from build123d import *

# Parameters (mm, degrees)
SKETCH1_R             = 1.2192
BOSS_EXTRUDE1_DEPTH   = 3.1242
BOSS_EXTRUDE1_2_DEPTH = 3.1242
BOSS_EXTRUDE1_3_DEPTH = 3.1242
BOSS_EXTRUDE1_4_DEPTH = 3.1242
BOSS_EXTRUDE2_START   = -1.27
SKETCH2_R             = 1.2192
BOSS_EXTRUDE2_DEPTH   = 1.27
SKETCH4_W             = 5.9436
SKETCH4_H             = 1.27
CUT_EXTRUDE1_DEPTH    = 1.27
FILLET1_DEPTH         = 3.1242
FILLET1_START         = 1.8542
FILLET1_2_DEPTH       = 1.27
BOSS_EXTRUDE3_DEPTH   = 1.27
FILLET2_R             = 0.889
FILLET3_R             = 0.889
FILLET5_R             = 1.27


with BuildPart() as part:
    # Sketch1 → Boss-Extrude1 (new body)
    with BuildSketch(Plane(origin=(0, 0, 0), x_dir=(1, 0, 0), z_dir=(0, 1, 0))):
        with BuildLine():
            Line((26.2382, 18.587486955), (26.2382, 12.248113045))
            ThreePointArc((26.2382, 12.248113045), (30.9753, 15.4178), (26.2382, 18.587486955))
        make_face()
        with Locations(Location((28.67025, 15.4178, 0), (0, 0, 270))):
            Circle(SKETCH1_R, mode=Mode.SUBTRACT)
    extrude(amount=BOSS_EXTRUDE1_DEPTH)



with BuildPart() as body_2:
    # Sketch1 → Boss-Extrude1 2 (new body)
    with BuildSketch(Plane(origin=(0, 0, 0), x_dir=(1, 0, 0), z_dir=(0, 1, 0))):
        with BuildLine():
            Line((-26.2382, 18.587486955), (-26.2382, 12.248113045))
            ThreePointArc((-26.2382, 12.248113045), (-30.9753, 15.4178), (-26.2382, 18.587486955))
        make_face()
        with Locations(Location((-28.67025, 15.4178, 0), (0, 0, 270))):
            Circle(SKETCH1_R, mode=Mode.SUBTRACT)
    extrude(amount=BOSS_EXTRUDE1_2_DEPTH)


with BuildPart() as body_3:
    # Sketch1 → Boss-Extrude1 3 (new body)
    with BuildSketch(Plane(origin=(0, 0, 0), x_dir=(1, 0, 0), z_dir=(0, 1, 0))):
        with BuildLine():
            Line((26.2382, -12.248113045), (26.2382, -18.587486955))
            ThreePointArc((26.2382, -18.587486955), (30.9753, -15.4178), (26.2382, -12.248113045))
        make_face()
        with Locations(Location((28.67025, -15.4178, 0), (0, 0, 270))):
            Circle(SKETCH1_R, mode=Mode.SUBTRACT)
    extrude(amount=BOSS_EXTRUDE1_3_DEPTH)


with BuildPart() as body_4:
    # Sketch1 → Boss-Extrude1 4 (new body)
    with BuildSketch(Plane(origin=(0, 0, 0), x_dir=(1, 0, 0), z_dir=(0, 1, 0))):
        with BuildLine():
            Line((-26.2382, -12.248113045), (-26.2382, -18.587486955))
            ThreePointArc((-26.2382, -18.587486955), (-30.9753, -15.4178), (-26.2382, -12.248113045))
        make_face()
        with Locations(Location((-28.67025, -15.4178, 0), (0, 0, 270))):
            Circle(SKETCH1_R, mode=Mode.SUBTRACT)
    extrude(amount=BOSS_EXTRUDE1_4_DEPTH)


with BuildPart() as part_1:
    add(part.part)

    add(body_2.part)  # Boss-Extrude2 merges body 2

    add(body_3.part)  # Boss-Extrude2 merges body 3

    add(body_4.part)  # Boss-Extrude2 merges body 4
    # Sketch2 → Boss-Extrude2 (add)
    with BuildSketch(Plane(origin=(0, 3.1242, 0), x_dir=(1, 0, 0), z_dir=(0, 1, 0)).offset(BOSS_EXTRUDE2_START)):
        with BuildLine():
            Line((-24.695157071, 17.3228), (24.695157071, 17.3228))
            ThreePointArc((24.695157071, 17.3228), (30.864949116, 16.280707319), (25.9842, 12.365278978))
            Line((25.9842, 12.365278978), (25.9842, -12.365278978))
            ThreePointArc((25.9842, -12.365278978), (30.879851828, -14.614386528), (27.5463, -18.8468))
            Line((27.5463, -18.8468), (-27.5463, -18.8468))
            ThreePointArc((-27.5463, -18.8468), (-30.879851828, -14.614386528), (-25.9842, -12.365278978))
            Line((-25.9842, -12.365278978), (-25.9842, 12.365278978))
            ThreePointArc((-25.9842, 12.365278978), (-30.864949116, 16.280707319), (-24.695157071, 17.3228))
        make_face()
        with Locations(Location((28.67025, -15.4178, 0), (0, 0, 270))):
            Circle(SKETCH2_R, mode=Mode.SUBTRACT)
        with Locations(Location((28.67025, 15.4178, 0), (0, 0, 270))):
            Circle(SKETCH2_R, mode=Mode.SUBTRACT)
        with Locations(Location((-28.67025, 15.4178, 0), (0, 0, 270))):
            Circle(SKETCH2_R, mode=Mode.SUBTRACT)
        with Locations(Location((-28.67025, -15.4178, 0), (0, 0, 270))):
            Circle(SKETCH2_R, mode=Mode.SUBTRACT)
    extrude(amount=BOSS_EXTRUDE2_DEPTH)

    # Sketch4 → Cut-Extrude1 (cut)
    with BuildSketch(Plane(origin=(0, 3.1242, 0), x_dir=(1, 0, 0), z_dir=(0, 1, 0))):
        with Locations((-10.8458, -18.2118)):
            Rectangle(SKETCH4_W, SKETCH4_H)
    extrude(amount=-CUT_EXTRUDE1_DEPTH, mode=Mode.SUBTRACT)

    # Fillet1: read off the stored shape, not the designer's step
    # Fillet1 outline → Fillet1 (add)
    with BuildSketch(Plane(origin=(0, 0, 0), x_dir=(1, 0, 0), z_dir=(0, 1, 0))):
        with BuildLine():
            Line((26.2382, 12.248113045), (26.2382, 9.318072184))
            ThreePointArc((26.2382, 9.318072184), (27.272818982, 11.08465566), (28.933486364, 12.281918148))
            ThreePointArc((28.933486364, 12.281918148), (27.58930418, 11.989069675), (26.2382, 12.248113045))
        make_face()
        with BuildLine():
            ThreePointArc((28.933486364, -12.281918148), (27.272818982, -11.08465566), (26.2382, -9.318072184))
            Line((26.2382, -9.318072184), (26.2382, -12.248113045))
            ThreePointArc((26.2382, -12.248113045), (27.58930418, -11.989069675), (28.933486364, -12.281918148))
        make_face()
        with BuildLine():
            Line((-26.2382, 9.318072184), (-26.2382, 12.248113045))
            ThreePointArc((-26.2382, 12.248113045), (-27.58930418, 11.989069675), (-28.933486364, 12.281918148))
            ThreePointArc((-28.933486364, 12.281918148), (-27.272818982, 11.08465566), (-26.2382, 9.318072184))
        make_face()
        with BuildLine():
            Line((-26.2382, -12.248113045), (-26.2382, -9.318072184))
            ThreePointArc((-26.2382, -9.318072184), (-27.272818982, -11.08465566), (-28.933486364, -12.281918148))
            ThreePointArc((-28.933486364, -12.281918148), (-27.58930418, -11.989069675), (-26.2382, -12.248113045))
        make_face()
    extrude(amount=FILLET1_DEPTH)

    # Fillet1 2 outline → Fillet1 2 (add)
    with BuildSketch(Plane(origin=(0, 0, 0), x_dir=(1, 0, 0), z_dir=(0, 1, 0)).offset(FILLET1_START)):
        with BuildLine():
            ThreePointArc((25.9842, 7.752311027), (26.048112355, 8.545425773), (26.2382, 9.318072184))
            Line((26.2382, 9.318072184), (26.2382, 12.248113045))
            ThreePointArc((26.2382, 12.248113045), (26.110004775, 12.304104924), (25.9842, 12.365278978))
            Line((25.9842, 12.365278978), (25.9842, 7.752311027))
        make_face()
        with BuildLine():
            ThreePointArc((26.2382, -9.318072184), (26.048112355, -8.545425773), (25.9842, -7.752311027))
            Line((25.9842, -7.752311027), (25.9842, -12.365278978))
            ThreePointArc((25.9842, -12.365278978), (26.110004775, -12.304104924), (26.2382, -12.248113045))
            Line((26.2382, -12.248113045), (26.2382, -9.318072184))
        make_face()
        with BuildLine():
            Line((-25.9842, -12.365278978), (-25.9842, -7.752311027))
            ThreePointArc((-25.9842, -7.752311027), (-26.048112355, -8.545425773), (-26.2382, -9.318072184))
            Line((-26.2382, -9.318072184), (-26.2382, -12.248113045))
            ThreePointArc((-26.2382, -12.248113045), (-26.110004775, -12.304104924), (-25.9842, -12.365278978))
        make_face()
        with BuildLine():
            Line((-24.695157071, 17.3228), (-22.726988846, 17.3228))
            ThreePointArc((-22.726988846, 17.3228), (-24.220374536, 17.553299795), (-25.574763619, 18.223345455))
            ThreePointArc((-25.574763619, 18.223345455), (-25.093280542, 17.813783418), (-24.695157071, 17.3228))
        make_face()
        with BuildLine():
            ThreePointArc((24.695157071, 17.3228), (25.093280542, 17.813783418), (25.574763619, 18.223345455))
            ThreePointArc((25.574763619, 18.223345455), (24.220374536, 17.553299795), (22.726988846, 17.3228))
            Line((22.726988846, 17.3228), (24.695157071, 17.3228))
        make_face()
        with BuildLine():
            ThreePointArc((-25.9842, 12.365278978), (-26.110004775, 12.304104924), (-26.2382, 12.248113045))
            Line((-26.2382, 12.248113045), (-26.2382, 9.318072184))
            ThreePointArc((-26.2382, 9.318072184), (-26.048112355, 8.545425773), (-25.9842, 7.752311027))
            Line((-25.9842, 7.752311027), (-25.9842, 12.365278978))
        make_face()
    extrude(amount=FILLET1_2_DEPTH)

    # Sketch7 → Boss-Extrude3 (add)
    with BuildSketch(Plane(origin=(0, 3.1242, 0), x_dir=(1, 0, 0), z_dir=(0, 1, 0))):
        Polygon((-7.874, -25.0444), (-7.874, -35.3314), (23.9649, -35.3314), (23.9649, -25.0444), (23.9649, -18.8468), (-7.874, -18.8468), align=None)
    extrude(amount=-BOSS_EXTRUDE3_DEPTH)

    # Fillet2
    fillet2_edges = [part_1.edges().sort_by_distance(p)[0] for p in [
        (-13.8176, 2.4892, 17.5768),
        (-7.874, 2.4892, 17.5768),
        (23.9649, 2.4892, 18.8468),
    ]]
    fillet(fillet2_edges, radius=FILLET2_R)

    # Fillet3
    fillet3_edges = [part_1.edges().sort_by_distance(p)[0] for p in [
        (-13.8176, 2.4892, 18.8468),
        (23.9649, 2.4892, 35.3314),
        (-7.874, 2.4892, 35.3314),
    ]]
    fillet(fillet3_edges, radius=FILLET3_R)

    # Fillet5
    # the kernel refuses this fillet: 1.27 mm, written as the material it takes off along each edge
    with BuildSketch(Plane(origin=(26.2382, -9.068202779, -9.318072184), x_dir=(0, 0, -1), z_dir=(0, 1, 0)), Plane(origin=(-26.2382, -9.068202779, 9.318072184), x_dir=(0, 0, 1), z_dir=(0, 1, 0))) as fillet5_piece_1:
        with BuildLine():
            CenterArc((3.627281111, -1.27), FILLET5_R, 90, 123.437045448)
            ThreePointArc((2.567476567, -1.969795919), (1.449146976, -0.769300527), (0, 0))
            Line((0, 0), (3.627281111, 0))
        make_face()
    extrude(amount=10.922402779, mode=Mode.SUBTRACT)
    with BuildSketch(Plane(origin=(26.2382, -9.068202779, 9.318072184), x_dir=(0, 0, 1), z_dir=(0, 1, 0)), Plane(origin=(-26.2382, -9.068202779, -9.318072184), x_dir=(0, 0, -1), z_dir=(0, 1, 0))) as fillet5_piece_2:
        with BuildLine():
            CenterArc((3.627281111, 1.27), FILLET5_R, 146.562954552, 123.437045448)
            ThreePointArc((2.567476567, 1.969795919), (1.449146976, 0.769300527), (0, 0))
            Line((0, 0), (3.627281111, 0))
        make_face()
    extrude(amount=10.922402779, mode=Mode.SUBTRACT)
    with BuildSketch(Plane(origin=(26.2382, -3.185360081, -18.587486955), x_dir=(0, 0, 1), z_dir=(0, 1, 0))) as fillet5_piece_3:
        with BuildLine():
            CenterArc((1.011023157, 1.27), FILLET5_R, 181.011154478, 88.988845522)
            ThreePointArc((-0.258779077, 1.247588235), (-0.187845593, 0.61166896), (0, 0))
            Line((0, 0), (1.011023157, 0))
        make_face()
    extrude(amount=5.039560081, mode=Mode.SUBTRACT)
    with BuildSketch(Plane(origin=(-26.2382, -3.185360081, 18.587486955), x_dir=(-0.9791579315799205, 0, 0.20310033240773342), z_dir=(0, 1, 0))) as fillet5_piece_4:
        with BuildLine():
            CenterArc((1.038191434, -1.247888766), FILLET5_R, 79.292837609, 88.988845522)
            Line((-0.205339139, -0.989951343), (0, 0))
            ThreePointArc((0, 0), (0.637072016, 0.059700333), (1.274144032, 0))
        make_face()
    extrude(amount=5.039560081, mode=Mode.SUBTRACT)
    with BuildSketch(Plane(origin=(-26.2382, -3.185360081, -18.587486955), x_dir=(0, 0, 1), z_dir=(0, 1, 0))) as fillet5_piece_5:
        with BuildLine():
            CenterArc((1.011023157, -1.27), FILLET5_R, 90, 88.988845522)
            ThreePointArc((-0.258779077, -1.247588235), (-0.187845593, -0.61166896), (0, 0))
            Line((0, 0), (1.011023157, 0))
        make_face()
    extrude(amount=5.039560081, mode=Mode.SUBTRACT)
    with BuildSketch(Plane(origin=(26.2382, -3.185360081, 18.587486955), x_dir=(0.9791579315799218, 0, 0.2031003324077264), z_dir=(0, 1, 0))) as fillet5_piece_6:
        with BuildLine():
            CenterArc((1.038191434, 1.247888766), FILLET5_R, 191.718316869, 88.988845522)
            Line((-0.205339139, 0.989951343), (0, 0))
            ThreePointArc((0, 0), (0.637072016, -0.059700333), (1.274144032, 0))
        make_face()
    extrude(amount=5.039560081, mode=Mode.SUBTRACT)


solid = part_1.part
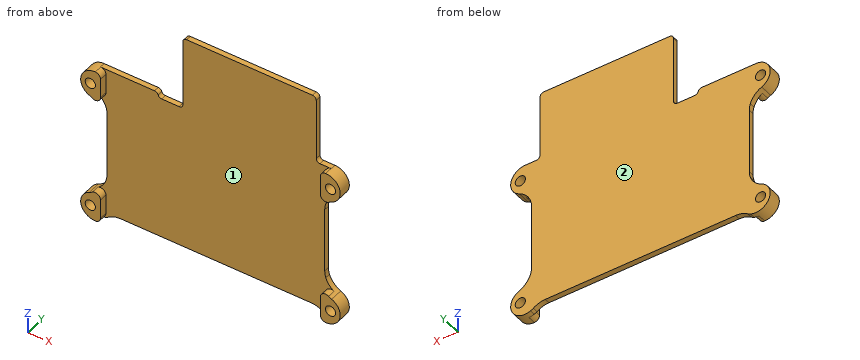
Geometry check sheet. Reference: the model listing, model coordinates, mm. Face numbers are marked on the shaded views. Round coordinates to 2 decimals unless told otherwise and drop trailing zeros. Order: outer loops, then holes, each group sorted by start corner. A loop starts at its lowest first (then second) coordinate and runs counter-clockwise, first axis right, second up. Notation, with made-up numbers: M -26,-19 L 6,-19 A15 ccw 6,8 Z; hole C -14,-16 d3. An arc over 180 degrees is marked long. Answer in a Markdown table with one row per item.
(1) Sectioned sample at B-B, the plane x = 19. Record the cut outline in (y, z), and give its area (3 significant figures).
Responses:
| item | result |
|---|---|
| outline | M 1.85,-17.32 L 3.12,-17.32 L 3.12,35.33 L 1.85,35.33 Z |
| area | 66.9 mm² |
(2) Draft check along X on the marked faces 1 and 2. Enter one of: released by +X, released by -X, zero draft, split by the parting line, or undercut.
Responses:
| item | result |
|---|---|
| face 1 | undercut |
| face 2 | zero draft |
(3) Sectioned sample at A-A, the plane y = 1. Record the cut outline in (x, z), and give its area (3 significant figures).
Responses:
| item | result |
|---|---|
| outline | M -28.93,-12.28 A3.43 ccw -27.49,-18.85 A1.27 ccw -26.24,-17.58 L -26.24,-12.95 A1.27 ccw -28.21,-11.89 A4.95 cw Z; M -28.93,12.28 A4.95 cw -28.21,11.89 A1.27 ccw -26.24,12.95 L -26.24,17.58 A1.27 ccw -27.49,18.85 A3.43 ccw Z; M 26.24,-17.58 A1.27 ccw 27.49,-18.85 A3.43 ccw 28.93,-12.28 A4.95 cw 28.21,-11.89 A1.27 ccw 26.24,-12.95 Z; M 26.24,12.95 A1.27 ccw 28.21,11.89 A4.95 cw 28.93,12.28 A3.43 ccw 27.49,18.85 A1.27 ccw 26.24,17.58 Z; hole C -28.67,-15.42 d2.44; hole C -28.67,15.42 d2.44; hole C 28.67,-15.42 d2.44; hole C 28.67,15.42 d2.44 |
| area | 90.8 mm² |
(4) Scan lines: probe 1 along X at (y, z) = (1.1, -16); probe 2 along Y at (x, z) = (9, 18.5); probe 3 along Z at (x, y) = (10, 2.1). Record each from-to range of solid material in increasing order. Write a range as from..to.
Responses:
| item | result |
|---|---|
| probe 1 | x = -30.93..-29.74, -27.6..-26.24, 26.24..27.6, 29.74..30.93 |
| probe 2 | y = 1.85..3.12 |
| probe 3 | z = -17.32..35.33 |
(5) Sectioned sample at C-C, the plane z = -6. Record the cut outline in (x, y), and give its area (3 significant figures).
Responses:
| item | result |
|---|---|
| outline | M -25.98,1.85 L 25.98,1.85 L 25.98,3.12 L -25.98,3.12 Z |
| area | 66.0 mm² |
(6) Go/stop test with flat-tipped pins: P1, Ø1, axis at x = 25.5, y = 2.5, coming from the +Z side; P2, Ø1, axis at x = 20.5, y = 0.5, coming from the +Z side; P3, Ø1, axis at y = 2.5, z = 25.5, coming from the +X side; P4, Ø1, axis at y = 2.5, z = 30, coming from the -X side. Record where each tip stops, or that it passes through.
Responses:
| item | result |
|---|---|
| P1 | stops at z = 18.85 |
| P2 | passes through |
| P3 | stops at x = 23.96 |
| P4 | stops at x = -7.87 |
